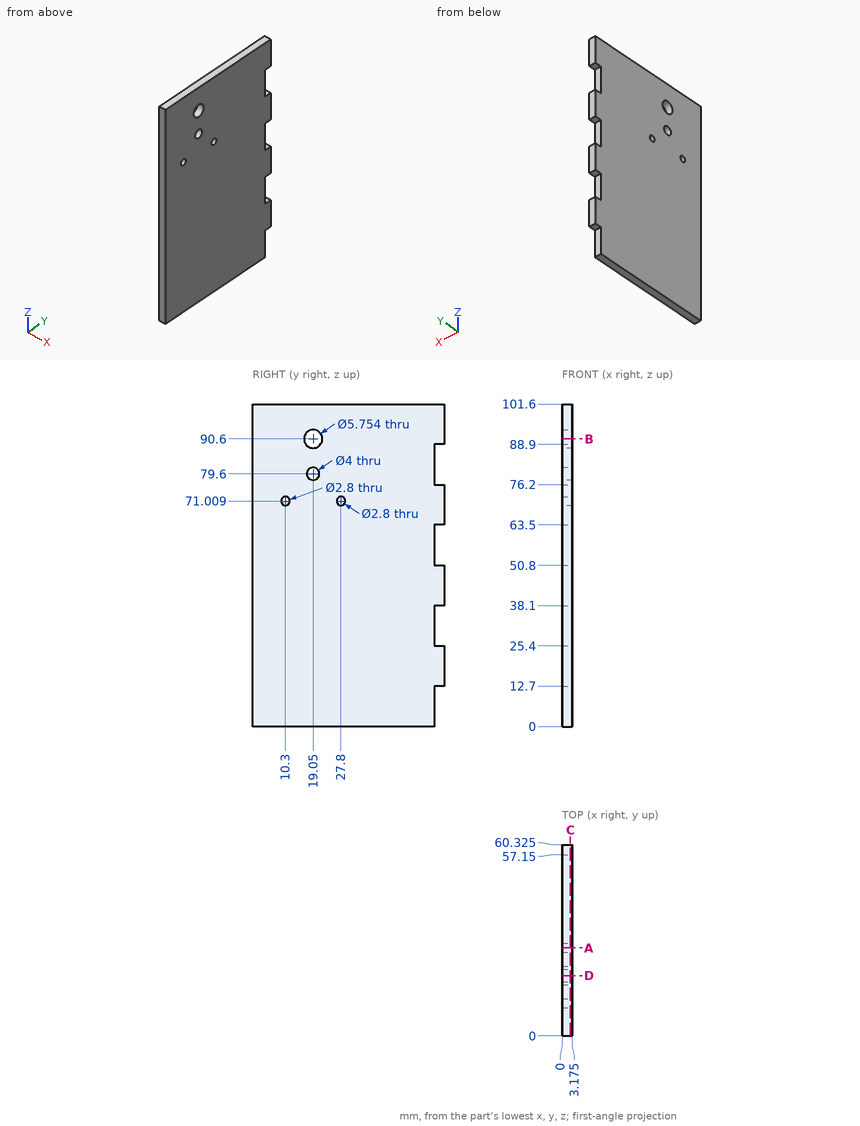
Can you work these out from the drawing? Everything is in mm from the part's minimum corner. Coordinates: 2 decimals unless noted, no trailing zeros. Loops run counter-clockwise (first coordinate to the right, second up) from the corner with the lowest first, then second, coordinate; pieces in that order, holes last. Notation, with made-up numbers: (35.5, 24.25) -> (84.5, 24.25) arc R19 ccw to (84.5, 55.25) -> close; hole circle Ø3 at (47, 6.5). An arc over 180 degrees is marked (long way). Return JSON: item names as keys, results as strings.
1) Will these pins go through, and if not, where does the flat tip stop? pin 1 (1 mm diameter, centred on x = 1, y = 58.5, fed in from -Z); pin 2 (1 mm diameter, centred on x = 1, z = 61.5, fed in from +Y); pin 3 (3.5 mm diameter, centred on y = 19.05, z = 90.6, fed in from +X).
Results below:
{"pin 1": "z = 12.7", "pin 2": "y = 57.15", "pin 3": "through"}
2) If we section it at C-C, the plane x = 2.55: Write out the boundary of the cut face in (y, z) (3 decimals).
Results below:
{"outline": "(0, 0) -> (57.15, 0) -> (57.15, 12.7) -> (60.325, 12.7) -> (60.325, 25.4) -> (57.15, 25.4) -> (57.15, 38.1) -> (60.325, 38.1) -> (60.325, 50.8) -> (57.15, 50.8) -> (57.15, 63.5) -> (60.325, 63.5) -> (60.325, 76.2) -> (57.15, 76.2) -> (57.15, 88.9) -> (60.325, 88.9) -> (60.325, 101.6) -> (0, 101.6) -> close; hole circle Ø2.8 at (10.3, 71.009); hole circle Ø5.754 at (19.05, 90.6); hole circle Ø4 at (19.05, 79.6); hole circle Ø2.8 at (27.8, 71.009)"}
3) If we section it at D-D, the plane y = 19.05: Write out the boundary of the cut face in (x, z) (3 decimals).
Results below:
{"outline": "(0, 0) -> (3.175, 0) -> (3.175, 77.6) -> (0, 77.6) -> close; (0, 81.6) -> (3.175, 81.6) -> (3.175, 87.723) -> (0, 87.723) -> close; (0, 93.477) -> (3.175, 93.477) -> (3.175, 101.6) -> (0, 101.6) -> close"}
4) If we section it at B-B, the plane z = 90.6: Write out the boundary of the cut face in (x, y) (3 decimals), then the cut area to 3 significant figures.
Results below:
{"outline": "(0, 0) -> (3.175, 0) -> (3.175, 16.173) -> (0, 16.173) -> close; (0, 21.927) -> (3.175, 21.927) -> (3.175, 60.325) -> (0, 60.325) -> close", "area": "173 mm²"}
5) I need wall thicknesses on line 1 (Y direction, x = 2.65, z = 71.5) (3 decimals); line 2 (Y direction, x = 1.45, z = 55.5); line 3 (Y direction, x = 1.9, z = 90.6) (3 decimals). Which ranges of each line are inside material? Lowest first, please. Write a range as from..to.
Results below:
{"line 1": "0..8.989, 11.611..26.489, 29.111..60.325", "line 2": "0..57.15", "line 3": "0..16.173, 21.927..60.325"}
6) If we section it at A-A, the plane y = 27.8: Write out the boundary of the cut face in (x, z) (3 decimals), then the cut area to 3 significant figures.
Results below:
{"outline": "(0, 0) -> (3.175, 0) -> (3.175, 69.609) -> (0, 69.609) -> close; (0, 72.409) -> (3.175, 72.409) -> (3.175, 101.6) -> (0, 101.6) -> close", "area": "314 mm²"}
